Model file for the job. Use its own axes, mm. A direction names the side the tool comes from. Coordinates: 2 decimals unless noted, no trailing zeros. Order: outer loops, then holes, each group sorted by start corner. A loop starts at its lowest first (then second) coordinate and runs counter-clockwise, first axis right, second up. Notation, with made-up numbers: (28, 43.5) - (49, 43.5) arc R31 cw to (49, 70.5) - close; hole circle Ø4 at (1, 21.5). An arc over 180 degrees is marked (long way). Put each result on its own line as item: value. Start each with the question number.
```python
from build123d import *

# Parameters (mm, degrees)
VERTICAL_BAR_DEPTH     = 15.875
CUT_CABLE_HOLDER_REACH = 17.875
SKETCH5_R              = 2.413
CUT_PIVOT_HOLE_REACH   = 17.875
SKETCH6_R              = 4.7117
CUT_EXTRUDE8_DEPTH     = 16.875
SLOT_CUT_DEPTH         = 7.62
SKETCH10_R             = 7.8105
CUT_EXTRUDE9_DEPTH     = 16.875
FILLET1_R              = 12.7


with BuildPart() as part:
    # Sketch3 → Vertical Bar (new body)
    with BuildSketch(Plane(origin=(0, 0, 0), x_dir=(0, 0, -1), z_dir=(1, 0, 0))):
        with BuildLine():
            Line((-12.7, -12.7), (12.7, -12.7))
            Line((12.7, -12.7), (8.138209265, 169.714598123))
            ThreePointArc((8.138209265, 169.714598123), (0, 189.170459445), (-8.138209265, 169.714598123))
            Line((-8.138209265, 169.714598123), (-12.7, -12.7))
        make_face()
    extrude(amount=-VERTICAL_BAR_DEPTH)

    # Sketch5 → Cut-Cable holder (cut, up to next)
    with BuildSketch(Plane(origin=(0, 0, 0), x_dir=(0, 0, -1), z_dir=(1, 0, 0)), mode=Mode.PRIVATE) as cut_cable_holder_sk1:
        with Locations((0, 50.8)):
            Circle(SKETCH5_R)
    cut_cable_holder_tool1 = extrude(cut_cable_holder_sk1.sketch, amount=-CUT_CABLE_HOLDER_REACH, mode=Mode.PRIVATE) & part.part
    add(cut_cable_holder_tool1.solids().sort_by_distance((0, 50.8, 0))[0], mode=Mode.SUBTRACT)
    # Sketch5 → Cut-Cable holder (cut, up to next)
    with BuildSketch(Plane(origin=(0, 0, 0), x_dir=(0, 0, -1), z_dir=(1, 0, 0)), mode=Mode.PRIVATE) as cut_cable_holder_sk2:
        with Locations((0, 63.5)):
            Circle(SKETCH5_R)
    cut_cable_holder_tool2 = extrude(cut_cable_holder_sk2.sketch, amount=-CUT_CABLE_HOLDER_REACH, mode=Mode.PRIVATE) & part.part
    add(cut_cable_holder_tool2.solids().sort_by_distance((0, 63.5, 0))[0], mode=Mode.SUBTRACT)
    # Sketch5 → Cut-Cable holder (cut, up to next)
    with BuildSketch(Plane(origin=(0, 0, 0), x_dir=(0, 0, -1), z_dir=(1, 0, 0)), mode=Mode.PRIVATE) as cut_cable_holder_sk3:
        with Locations((0, 76.2)):
            Circle(SKETCH5_R)
    cut_cable_holder_tool3 = extrude(cut_cable_holder_sk3.sketch, amount=-CUT_CABLE_HOLDER_REACH, mode=Mode.PRIVATE) & part.part
    add(cut_cable_holder_tool3.solids().sort_by_distance((0, 76.2, 0))[0], mode=Mode.SUBTRACT)
    # Sketch5 → Cut-Cable holder (cut, up to next)
    with BuildSketch(Plane(origin=(0, 0, 0), x_dir=(0, 0, -1), z_dir=(1, 0, 0)), mode=Mode.PRIVATE) as cut_cable_holder_sk4:
        with Locations((0, 88.9)):
            Circle(SKETCH5_R)
    cut_cable_holder_tool4 = extrude(cut_cable_holder_sk4.sketch, amount=-CUT_CABLE_HOLDER_REACH, mode=Mode.PRIVATE) & part.part
    add(cut_cable_holder_tool4.solids().sort_by_distance((0, 88.9, 0))[0], mode=Mode.SUBTRACT)
    # Sketch5 → Cut-Cable holder (cut, up to next)
    with BuildSketch(Plane(origin=(0, 0, 0), x_dir=(0, 0, -1), z_dir=(1, 0, 0)), mode=Mode.PRIVATE) as cut_cable_holder_sk5:
        with Locations((0, 101.6)):
            Circle(SKETCH5_R)
    cut_cable_holder_tool5 = extrude(cut_cable_holder_sk5.sketch, amount=-CUT_CABLE_HOLDER_REACH, mode=Mode.PRIVATE) & part.part
    add(cut_cable_holder_tool5.solids().sort_by_distance((0, 101.6, 0))[0], mode=Mode.SUBTRACT)
    # Sketch5 → Cut-Cable holder (cut, up to next)
    with BuildSketch(Plane(origin=(0, 0, 0), x_dir=(0, 0, -1), z_dir=(1, 0, 0)), mode=Mode.PRIVATE) as cut_cable_holder_sk6:
        with Locations((0, 114.3)):
            Circle(SKETCH5_R)
    cut_cable_holder_tool6 = extrude(cut_cable_holder_sk6.sketch, amount=-CUT_CABLE_HOLDER_REACH, mode=Mode.PRIVATE) & part.part
    add(cut_cable_holder_tool6.solids().sort_by_distance((0, 114.3, 0))[0], mode=Mode.SUBTRACT)
    # Sketch5 → Cut-Cable holder (cut, up to next)
    with BuildSketch(Plane(origin=(0, 0, 0), x_dir=(0, 0, -1), z_dir=(1, 0, 0)), mode=Mode.PRIVATE) as cut_cable_holder_sk7:
        with Locations((0, 127)):
            Circle(SKETCH5_R)
    cut_cable_holder_tool7 = extrude(cut_cable_holder_sk7.sketch, amount=-CUT_CABLE_HOLDER_REACH, mode=Mode.PRIVATE) & part.part
    add(cut_cable_holder_tool7.solids().sort_by_distance((0, 127, 0))[0], mode=Mode.SUBTRACT)
    # Sketch5 → Cut-Cable holder (cut, up to next)
    with BuildSketch(Plane(origin=(0, 0, 0), x_dir=(0, 0, -1), z_dir=(1, 0, 0)), mode=Mode.PRIVATE) as cut_cable_holder_sk8:
        with Locations((0, 139.7)):
            Circle(SKETCH5_R)
    cut_cable_holder_tool8 = extrude(cut_cable_holder_sk8.sketch, amount=-CUT_CABLE_HOLDER_REACH, mode=Mode.PRIVATE) & part.part
    add(cut_cable_holder_tool8.solids().sort_by_distance((0, 139.7, 0))[0], mode=Mode.SUBTRACT)
    # Sketch5 → Cut-Cable holder (cut, up to next)
    with BuildSketch(Plane(origin=(0, 0, 0), x_dir=(0, 0, -1), z_dir=(1, 0, 0)), mode=Mode.PRIVATE) as cut_cable_holder_sk9:
        with Locations((0, 158.75)):
            Circle(SKETCH5_R)
    cut_cable_holder_tool9 = extrude(cut_cable_holder_sk9.sketch, amount=-CUT_CABLE_HOLDER_REACH, mode=Mode.PRIVATE) & part.part
    add(cut_cable_holder_tool9.solids().sort_by_distance((0, 158.75, 0))[0], mode=Mode.SUBTRACT)
    # Sketch5 → Cut-Cable holder (cut, up to next)
    with BuildSketch(Plane(origin=(0, 0, 0), x_dir=(0, 0, -1), z_dir=(1, 0, 0)), mode=Mode.PRIVATE) as cut_cable_holder_sk10:
        with Locations((0, 38.1)):
            Circle(SKETCH5_R)
    cut_cable_holder_tool10 = extrude(cut_cable_holder_sk10.sketch, amount=-CUT_CABLE_HOLDER_REACH, mode=Mode.PRIVATE) & part.part
    add(cut_cable_holder_tool10.solids().sort_by_distance((0, 38.1, 0))[0], mode=Mode.SUBTRACT)

    # Sketch6 → Cut-Pivot hole (cut, up to next)
    with BuildSketch(Plane(origin=(0, 0, 0), x_dir=(0, 0, -1), z_dir=(1, 0, 0)), mode=Mode.PRIVATE) as cut_pivot_hole_sk1:
        Circle(SKETCH6_R)
    cut_pivot_hole_tool1 = extrude(cut_pivot_hole_sk1.sketch, amount=-CUT_PIVOT_HOLE_REACH, mode=Mode.PRIVATE) & part.part
    add(cut_pivot_hole_tool1.solids().sort_by_distance((0, 0, 0))[0], mode=Mode.SUBTRACT)

    # Sketch8 → Cut-Extrude8 (cut, through all)
    with BuildSketch(Plane(origin=(0, 0, 0), x_dir=(0, 0, -1), z_dir=(1, 0, 0))):
        with BuildLine():
            Line((-12.382400735, 0), (-12.7, -12.7))
            Line((-12.7, -12.7), (12.7, -12.7))
            Line((12.7, -12.7), (12.382400735, 0))
            ThreePointArc((12.382400735, 0), (0, -12.382400735), (-12.382400735, 0))
        make_face()
    extrude(amount=-CUT_EXTRUDE8_DEPTH, mode=Mode.SUBTRACT)

    # Sketch9 → Slot Cut (cut)
    with BuildSketch(Plane.ZY.offset(15.875)):
        with BuildLine():
            Line((-6.35, 140.97), (-6.35, 31.75))
            ThreePointArc((-6.35, 31.75), (0, 25.4), (6.35, 31.75))
            Line((6.35, 31.75), (6.35, 140.97))
            ThreePointArc((6.35, 140.97), (0, 147.32), (-6.35, 140.97))
        make_face()
    extrude(amount=-SLOT_CUT_DEPTH, mode=Mode.SUBTRACT)

    # Sketch10 → Cut-Extrude9 (cut, through all)
    with BuildSketch(Plane(origin=(0, 0, 0), x_dir=(0, 0, -1), z_dir=(1, 0, 0))):
        with Locations((0, 177.8)):
            Circle(SKETCH10_R)
    extrude(amount=-CUT_EXTRUDE9_DEPTH, mode=Mode.SUBTRACT)

    # Fillet1
    fillet1_edges = [part.edges().sort_by_distance(p)[0] for p in [
        (-7.9375, 169.714598123, 8.138209265),
        (-7.9375, 169.714598123, -8.138209265),
    ]]
    fillet(fillet1_edges, radius=FILLET1_R)


solid = part.part
```
Item 1: 3-axis set-ups, long thin cutter, end or side, ignore diameter. For faces 5 (the face through (-7.826, 156.394, 0.523)), 6 (the face through (-8.255, 87, -3)): which of +Z, -Z, +X, -X, +Y, -Y reach the whole face in a straight line?
Item 2: Slice it at C-C, the plane x = -10.25. Give the cut face in (y, z), plus the area to 3 significant figures.
Item 3: Slice it at B-B, the plane x = -2.75. Give the number of separate pieces and of enclosed holes in the cut face, plus the area to 3 significant figures.
Item 4: Wall check: line 1 along Y through (x, z) = (-6.5, -4); line 2 along Z through (x, y) = (-14.25, 98.5); line 3 along X through (y, z) = (134.5, -4.5) (3 decimals). Give the ranges that are in metal, low to high.
Item 5: Flat gauge pins, fed straight in: pin 1 Ø10 at (y, z) = (63.5, 3.5) entering from +X; pin 2 Ø6.5 at (y, z) = (38.1, 0) entering from -X (3 decimals); pin 3 Ø3 at (x, z) = (-5, -6) entering from +Y; pin 4 Ø5 at (x, y) = (-6.5, 138) entering from +Z. Where does each tip first touch, or does it go through?
Item 6: Pull direction Z, two halves, no side cores. Call faces 1 (the face through (-4.07, 40.135, -1.297)), 2 (the face through (-12.1, 25.4, -0.1)), 3 (the face through (-8.049, 168.816, 8.616)), 4 (the face through (-8.05, 168.91, -8.64)): pulls with the +Z half, pulls with the -Z half, needs draft (parallel to the pull), parting line crosses it, or undercut.
Item 7: Slice it at A-A, the plane y = 114.3. Give the cut face in (x, z) (3 decimals).
Here are the results:
1. face 5: +X, -X
1. face 6: -X
2. outline: (0, -12.38) - (165.43, -8.25) arc R12.7 cw to (172.06, -9.92) arc R11.43 ccw (long way) to (172.06, 9.92) arc R12.7 cw to (165.43, 8.25) - (0, 12.38) arc R12.38 ccw to start; hole circle Ø9.42 at (0, 0); hole (31.75, -6.35) - (140.97, -6.35) arc R6.35 ccw to (140.97, 6.35) - (31.75, 6.35) arc R6.35 ccw to start; hole circle Ø4.83 at (158.75, 0); hole circle Ø15.62 at (177.8, 0)
2. area: 2,310 mm^2
3. separate pieces: 1
3. enclosed holes: 12
3. area: 3,650 mm^2
4. line 1: y = -11.72 to -2.49, 2.49 to 171.09, 184.51 to 188.45
4. line 2: z = -9.92 to -6.35, 6.35 to 9.92
4. line 3: x = -8.255 to 0
5. pin 1: stops at x = 0
5. pin 2: stops at x = -8.255
5. pin 3: stops at y = 188.25
5. pin 4: stops at z = 8.99
6. face 1: undercut
6. face 2: undercut
6. face 3: pulls with the +Z half
6. face 4: pulls with the -Z half
7. outline: (-15.875, -9.524) - (0, -9.524) - (0, -2.413) - (-8.255, -2.413) - (-8.255, -6.35) - (-15.875, -6.35) - close; (-15.875, 6.35) - (-8.255, 6.35) - (-8.255, 2.413) - (0, 2.413) - (0, 9.524) - (-15.875, 9.524) - close
